```python
from build123d import *


with BuildPart() as part:
    # Body: sweep along a path in PathSke
    with BuildLine(Plane(origin=(1.207969362, 1.807969362, 0), x_dir=(0, 1, 0), z_dir=(0, 0, 1))) as body_path:
        Line((-0.357969362, -30.192030638), (-0.357969362, -5.192030638))
        ThreePointArc((-0.357969362, -5.192030638), (-0.201939729, -4.407742914), (0.242387718, -3.742892857))
        ThreePointArc((0.242387718, -3.742892857), (-1.807969362, 1.207969362), (-3.858326443, -3.742892857))
        ThreePointArc((-3.858326443, -3.742892857), (-3.413998995, -4.407742914), (-3.257969362, -5.192030638))
        Line((-3.257969362, -5.192030638), (-3.257969362, -33.392030638))
    # SectionSke → Body (sweep)
    with BuildSketch(Plane(origin=(31.4, 0.15, 0.15), x_dir=(0, 1, 0), z_dir=(1, 0, 0))):
        with BuildLine():
            Line((-0.15, -1.6), (-0.15, 1.3))
            ThreePointArc((-0.15, 1.3), (1.3, -0.15), (-0.15, -1.6))
        make_face()
    sweep(path=body_path.line)


solid = part.part
```
Work out the finished part from the listing and answer in its coordinate system (mm). A direction names the side the tool comes from. Round coordinates to 2 decimals unless told otherwise and drop trailing zeros. Write each loop counter-clockwise with the first axis right and the second up, starting at its lowest first coordinate (ties: lowest second). Pieces come first, ordered by that corner, then holes. Notation, with made-up numbers: (-7.5, 25.5) - (42.5, 25.5) arc R11 ccw to (42.5, 36.5) - close; hole circle Ø3 at (-7, -12.75). An arc over 180 degrees is marked (long way). Return JSON: item names as keys, results as strings. Group by question number.
Q1. The part is cut by section B-B on x = 13. Write down the section's boundary in (y, z).
Q2. For faces 1 (the flat face through (34.6, -1, 0)), 2 (the flat face through (31.4, 1, 0)), 3 (the cylindrical face through (18.72, 1.45, 0.03)), 4 (the cylindrical face through (20.7, -1.45, 0.03)), determine the directions among +Z, -Z, +X, -X, +Y, -Y from which every point of the face is accessible in a straight line to the end or side of a thin tool.
Q3. Each of these flat-tipped pins is pushed along its axis until it touches: pin 1 Ø3 at (x, y) = (26, 2) entering from +Z; pin 2 Ø2.5 at (x, y) = (2.9, 0) entering from -Z; pin 3 Ø2 at (x, y) = (31, -0.5) entering from +Z. Where does it stop, or does it pass through?
Solved:
{
 "1": {"outline": "circle Ø2.9 at (0, 0)"},
 "2": {"face 1": "+Z, -Z, +X, +Y, -Y", "face 2": "+Z, -Z, +X, +Y", "face 3": "+X, +Y", "face 4": "+X, -Y"},
 "3": {"pin 1": "z = 1.36", "pin 2": "through", "pin 3": "z = 1.45"}
}
